CAD build for the part. Positions are in the model's coordinates, mm. Face numbers are marked on the shaded views. A direction names the side the tool comes from. Round coordinates to 2 decimals unless told otherwise and drop trailing zeros. Loops run counter-clockwise (first coordinate to the right, second up) from the corner with the lowest first, then second, coordinate; pieces in that order, holes last.
from build123d import *

# Parameters (mm, degrees)
CUT_EXTRUDE_5_REACH      = 12
SKETCH_2_R               = 2.5
SKETCH_2_R_2             = 2
CUT_EXTRUDE_8_DEPTH      = 0.8
CHAMFER_1_SIZE           = 0.2
CHAMFER_2_SIZE           = 0.1
SKETCH_4_R               = 3.825
CUT_EXTRUDE_9_DEPTH      = 0.25
CUT_EXTRUDE_9_DEPTH_BACK = 0.25


with BuildPart() as part:
    # Эскиз1 → Повернуть1 (revolve)
    with BuildSketch(Plane.XY):
        Polygon((0, 0), (0, 2.5), (1.6, 2.5), (1.6, 1.1), (1.7, 1), (7.1, 1), (7.15, 0.95), (10, 0.95), (10, 0), align=None)
    revolve(axis=Axis((0, 0, 0), (-1, 0, 0)))

    # Эскиз2 → Вырез-Вытянуть5 (cut, up to next)
    with BuildSketch(Plane.ZY, mode=Mode.PRIVATE) as cut_extrude_5_sk1:
        Circle(SKETCH_2_R)
        with Locations((0, -0.25)):
            Circle(SKETCH_2_R_2, mode=Mode.SUBTRACT)
    cut_extrude_5_tool1 = extrude(cut_extrude_5_sk1.sketch, amount=-CUT_EXTRUDE_5_REACH, mode=Mode.PRIVATE) & part.part
    add(cut_extrude_5_tool1.solids().sort_by_distance((0, 0, -2.429289))[0], mode=Mode.SUBTRACT)

    # Эскиз3 → Вырез-Вытянуть8 (cut)
    with BuildSketch(Plane(origin=(10, 0, 0), x_dir=(0, 0, -1), z_dir=(1, 0, 0))):
        with BuildLine():
            ThreePointArc((0.15, 0.938083152), (0, 0.95), (-0.15, 0.938083152))
            Line((-0.15, 0.938083152), (-0.15, -0.938083152))
            ThreePointArc((-0.15, -0.938083152), (0, -0.95), (0.15, -0.938083152))
            Line((0.15, -0.938083152), (0.15, 0.938083152))
        make_face()
    extrude(amount=-CUT_EXTRUDE_8_DEPTH, mode=Mode.SUBTRACT)

    # Фаска1
    chamfer_1_edges = [part.edges().sort_by_distance(p)[0] for p in [
        (10, 0, 0.95),
        (10, 0, -0.95),
    ]]
    chamfer(chamfer_1_edges, length=CHAMFER_1_SIZE)

    # Фаска2
    chamfer_2_edges = [part.edges().sort_by_distance(p)[0] for p in [
        (0, -0.25, -2),
        (1.6, -0.25, -2),
    ]]
    chamfer(chamfer_2_edges, length=CHAMFER_2_SIZE)

    # Эскиз4 → Вырез-Вытянуть9 (cut, two sides)
    with BuildSketch(Plane.XY) as cut_extrude_9_sk:
        with Locations((-3.425, -0.25)):
            Circle(SKETCH_4_R)
    extrude(amount=CUT_EXTRUDE_9_DEPTH, mode=Mode.SUBTRACT)
    extrude(cut_extrude_9_sk.sketch, amount=-CUT_EXTRUDE_9_DEPTH_BACK, mode=Mode.SUBTRACT)


solid = part.part
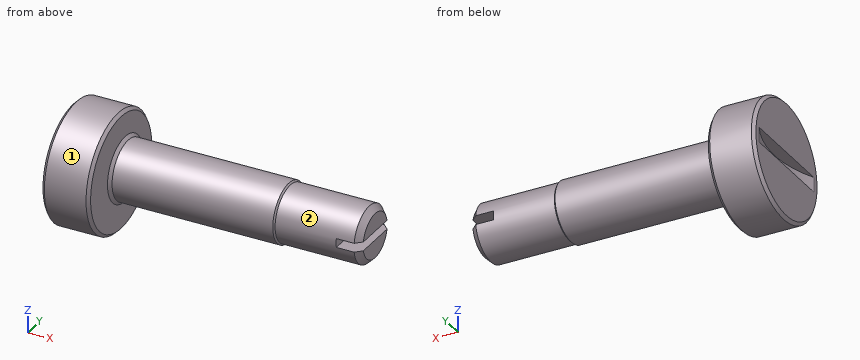
Item 1: 3-axis set-ups, long thin cutter, end or side, ignore diameter. For the marked faces 1 and 2: which of +Z, -Z, +X, -X, +Y, -Y reach the whole face in a straight line?
Verdict:
face 1: +X, -X
face 2: +X
Item 2: Cut at C-C (x = 4.25). List the corners of the cut face in (y, z).
Verdict:
outline: circle Ø2 at (0, 0)
Item 3: Cut at B-B (x = 9). List the corners of the cut face in (y, z).
Verdict:
outline: circle Ø1.9 at (0, 0)
Item 4: Cut at A-A (z = 0). List the corners of the cut face in (x, y) (3 decimals).
Verdict:
outline: (0, -2.15) - (0.1, -2.25) - (1.5, -2.25) - (1.6, -2.15) - (1.6, -1.1) - (1.7, -1) - (7.1, -1) - (7.15, -0.95) - (9.2, -0.95) - (9.2, 0.95) - (7.15, 0.95) - (7.1, 1) - (1.7, 1) - (1.6, 1.1) - (1.6, 1.65) - (1.5, 1.75) - (0.1, 1.75) - (0, 1.65) - (0, 1.453) arc R3.825 cw to (0, -1.953) - close
Item 5: Flat gauge pin, fed straight in: P1, Ø1.5, axis at x = 2, y = 1, coming from the -Z side. Where does the tip first touch, or does it go through?
Verdict:
P1: stops at z = -1.88
Item 6: Wall check: L1, parallel to Y at x = 8, z = -0.15; L2, parallel to Z at x = 5.25, y = 0. Give the ranges that are in metal, low to high.
Verdict:
L1: y = -0.94 to 0.94
L2: z = -1 to 1
